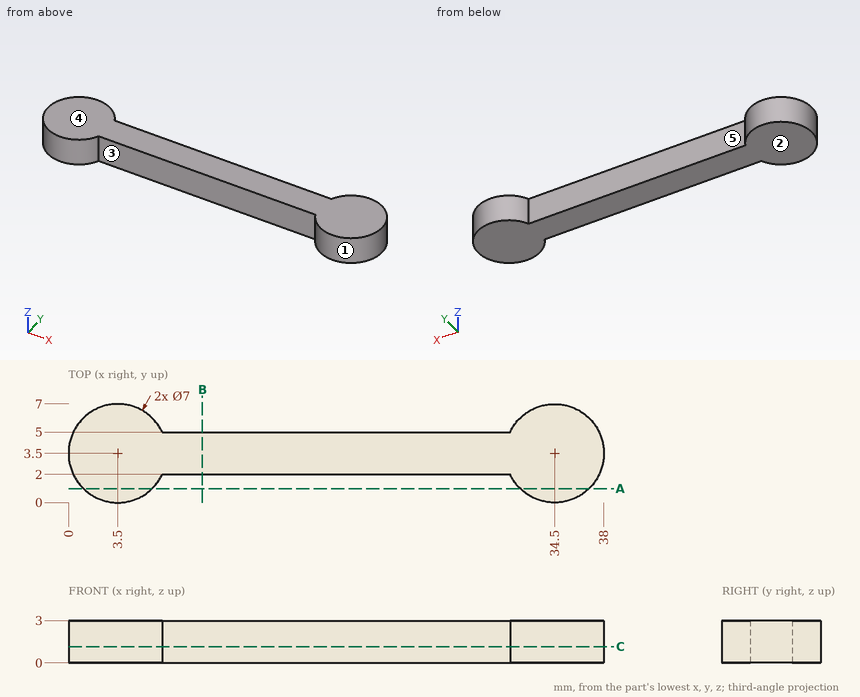
Geometry: see drawing. Coordinates: mm, zero at the bounding-box minimum. A direction names the side the tool comes from. Round coordinates to 2 decimals unless told otherwise and drop trailing zeros. Write each loop counter-clockwise with the first axis right and the second up, starting at its lowest first coordinate (ties: lowest second). Pieces come first, ordered by that corner, then holes. Notation, with made-up numbers: (-32.75, -2) -> (-0.75, -2) arc R14 ccw to (-0.75, 5) -> close; hole circle Ø11 at (-5, -33.75). An arc over 180 degrees is marked (long way). Answer as CSV lines item,"result".
1. Section C-C (z = 1.15). Return the cut outline in (x, y), plus the area to 3 significant figures.
Geometry says:
outline,"(6.66, 2) -> (31.34, 2) arc R3.5 ccw (long way) to (31.34, 5) -> (6.66, 5) arc R3.5 ccw (long way) to start"
area,"150 mm^2"
2. Reachability of the marked faces 4 and 5 from +Z, -Z, +X, -X, +Y, -Y: full face, straight path, thin tool, end or side. Return the list, or none.
Geometry says:
face 4,"+Z, +X, -X, +Y, -Y"
face 5,"+Z, -Z, +Y"
3. Ray query, L1, parallel to Y at x = 10.5, z = 0.75; L2, parallel to X at y = 6, z = 1.9; L3, parallel to X at y = 1.25, z = 2.8. Return the intervals inside material, ascending. Write a range as [from, to].
Geometry says:
L1,"y = [2, 5]"
L2,"x = [1.05, 5.95], [32.05, 36.95]"
L3,"x = [0.82, 6.18], [31.82, 37.18]"
4. Mould query, pull axis X, two halves, no side actions, for the marked faces 1, 2 and 3. Classes: +X half, -X half, draft (parallel to the pull), parting line (faces both ways), or undercut.
Geometry says:
face 1,"undercut"
face 2,"draft"
face 3,"undercut"
5. Section B-B (x = 9.5). Return the cut outline in (y, z).
Geometry says:
outline,"(2, 0) -> (5, 0) -> (5, 3) -> (2, 3) -> close"
6. Contact query for a flat-ended pin moving along its axis: P1, Ø0.9, axis at x = 14.5, z = 1, coming from the -Y side. Output: stop coordinate, or through.
Geometry says:
P1,"stops at y = 2"
7. Section A-A (y = 1). Return the cut outline in (x, z), plus the area to 3 significant figures.
Geometry says:
outline,"(1.05, 0) -> (5.95, 0) -> (5.95, 3) -> (1.05, 3) -> close; (32.05, 0) -> (36.95, 0) -> (36.95, 3) -> (32.05, 3) -> close"
area,"29.4 mm^2"
